from build123d import *

# Parameters (mm, degrees)
SKETCH1_W           = 30
SKETCH1_H           = 30
SKETCH1_R           = 2.65
BOSS_EXTRUDE1_DEPTH = 31
SKETCH2_W           = 30
SKETCH2_H           = 30
BOSS_EXTRUDE2_DEPTH = 10
BOSS_EXTRUDE3_DEPTH = 5
CHAMFER1_SIZE       = 5
CUT_EXTRUDE1_REACH  = 37
SKETCH4_R           = 1.6


with BuildPart() as part:
    # Sketch1 → Boss-Extrude1 (new body)
    with BuildSketch(Plane.XY):
        Rectangle(SKETCH1_W, SKETCH1_H)
        Circle(SKETCH1_R, mode=Mode.SUBTRACT)
    extrude(amount=BOSS_EXTRUDE1_DEPTH)

    # Sketch2 → Boss-Extrude2 (add)
    with BuildSketch(Plane.XY.offset(31)):
        Rectangle(SKETCH2_W, SKETCH2_H)
    extrude(amount=BOSS_EXTRUDE2_DEPTH)

    # Sketch3 → Boss-Extrude3 (add)
    with BuildSketch(Plane(origin=(0, 15, 0), x_dir=(1, 0, 0), z_dir=(0, 1, 0))):
        Polygon((0, 0), (-25, 0), (-25, -50), (25, -50), (25, 0), align=None)
    extrude(amount=BOSS_EXTRUDE3_DEPTH)

    # Chamfer1
    chamfer1_edges = [part.edges().sort_by_distance(p)[0] for p in [
        (15, -15, 20.5),
        (-15, -15, 20.5),
    ]]
    chamfer(chamfer1_edges, length=CHAMFER1_SIZE)

    # Sketch4 → Cut-Extrude1 (cut, up to next)
    with BuildSketch(Plane(origin=(0, 20, 0), x_dir=(1, 0, 0), z_dir=(0, 1, 0)), mode=Mode.PRIVATE) as cut_extrude1_sk1:
        with Locations((-20, -5)):
            Circle(SKETCH4_R)
    cut_extrude1_tool1 = extrude(cut_extrude1_sk1.sketch, amount=-CUT_EXTRUDE1_REACH, mode=Mode.PRIVATE) & part.part
    add(cut_extrude1_tool1.solids().sort_by_distance((-20, 20, 5))[0], mode=Mode.SUBTRACT)
    # Sketch4 → Cut-Extrude1 (cut, up to next)
    with BuildSketch(Plane(origin=(0, 20, 0), x_dir=(1, 0, 0), z_dir=(0, 1, 0)), mode=Mode.PRIVATE) as cut_extrude1_sk2:
        with Locations((20, -5)):
            Circle(SKETCH4_R)
    cut_extrude1_tool2 = extrude(cut_extrude1_sk2.sketch, amount=-CUT_EXTRUDE1_REACH, mode=Mode.PRIVATE) & part.part
    add(cut_extrude1_tool2.solids().sort_by_distance((20, 20, 5))[0], mode=Mode.SUBTRACT)
    # Sketch4 → Cut-Extrude1 (cut, up to next)
    with BuildSketch(Plane(origin=(0, 20, 0), x_dir=(1, 0, 0), z_dir=(0, 1, 0)), mode=Mode.PRIVATE) as cut_extrude1_sk3:
        with Locations((20, -45)):
            Circle(SKETCH4_R)
    cut_extrude1_tool3 = extrude(cut_extrude1_sk3.sketch, amount=-CUT_EXTRUDE1_REACH, mode=Mode.PRIVATE) & part.part
    add(cut_extrude1_tool3.solids().sort_by_distance((20, 20, 45))[0], mode=Mode.SUBTRACT)
    # Sketch4 → Cut-Extrude1 (cut, up to next)
    with BuildSketch(Plane(origin=(0, 20, 0), x_dir=(1, 0, 0), z_dir=(0, 1, 0)), mode=Mode.PRIVATE) as cut_extrude1_sk4:
        with Locations((-20, -45)):
            Circle(SKETCH4_R)
    cut_extrude1_tool4 = extrude(cut_extrude1_sk4.sketch, amount=-CUT_EXTRUDE1_REACH, mode=Mode.PRIVATE) & part.part
    add(cut_extrude1_tool4.solids().sort_by_distance((-20, 20, 45))[0], mode=Mode.SUBTRACT)


solid = part.part
For this review, take the finished solid that the model builds, in its own axes (mm). A direction names the side the tool comes from. Coordinates: 2 decimals unless noted, no trailing zeros. Loops run counter-clockwise (first coordinate to the right, second up) from the corner with the lowest first, then second, coordinate; pieces in that order, holes last. Notation, with made-up numbers: (6, 1) - (38, 1) arc R26 ccw to (38, 34) - close; hole circle Ø7 at (-28, 10.5). An arc over 180 degrees is marked (long way). Return JSON: item names as keys, results as strings.
Item 1: Take a section at D-D (y = 0). Give the boundary of the cut face in (x, z).
Determined:
{"outline": "(-15, 0) - (-2.65, 0) - (-2.65, 31) - (2.65, 31) - (2.65, 0) - (15, 0) - (15, 41) - (-15, 41) - close"}
Item 2: For faces 4 (the flat face through (0, 0, 31)), 5 (the flat face through (0, 0, 41)), 6 (the flat face through (-15, 2, 20)), list the 3-axis set-ups (+Z, -Z, +X, -X, +Y, -Y) from which the entire face can be reached by the end or side of a thin tool; tool diameter is ignored.
Determined:
{"face 4": "-Z", "face 5": "+Z, +X, -X, -Y", "face 6": "+Z, -Z, -X, -Y"}
Item 3: Take a section at A-A (z = 5). Give the boundary of the cut face in (x, y).
Determined:
{"outline": "(-25, 15) - (-21.6, 15) - (-21.6, 20) - (-25, 20) - close; (-18.4, 15) - (-15, 15) - (-15, -10) - (-10, -15) - (10, -15) - (15, -10) - (15, 15) - (18.4, 15) - (18.4, 20) - (-18.4, 20) - close; (21.6, 15) - (25, 15) - (25, 20) - (21.6, 20) - close; hole circle Ø5.3 at (0, 0)"}
Item 4: For line 1 (X direction, y = 17.8, z = 5); line 2 (Z direction, x = -20, y = 16.85); line 3 (Z direction, x = 1, y = 11), list the stretches that pass through material, from the lowest coordinate up.
Determined:
{"line 1": "x = -25 to -21.6, -18.4 to 18.4, 21.6 to 25", "line 2": "z = 0 to 3.4, 6.6 to 43.4, 46.6 to 50", "line 3": "z = 0 to 41"}
Item 5: Take a section at C-C (z = 23.5). Give the boundary of the cut face in (x, y), then the cut area to 3 significant figures.
Determined:
{"outline": "(-25, 15) - (-15, 15) - (-15, -10) - (-10, -15) - (10, -15) - (15, -10) - (15, 15) - (25, 15) - (25, 20) - (-25, 20) - close; hole circle Ø5.3 at (0, 0)", "area": "1,100 mm2"}
Item 6: Mouldability with a two-part tool opening along Z and no side actions: class faces 1 (the flat face through (0, 17, 50)), 2 (the cylindrical face through (18.73, 17.54, 45.97)), 3 (the flat face through (-25, 17, 25)) as pulls with the +Z half, pulls with the -Z half, needs draft (parallel to the pull), parting line crosses it, or undercut.
Determined:
{"face 1": "pulls with the +Z half", "face 2": "undercut", "face 3": "needs draft"}
Item 7: Take a section at B-B (x = 20). Give the boundary of the cut face in (y, z), then the cut area to 3 significant figures.
Determined:
{"outline": "(15, 0) - (20, 0) - (20, 3.4) - (15, 3.4) - close; (15, 6.6) - (20, 6.6) - (20, 43.4) - (15, 43.4) - close; (15, 46.6) - (20, 46.6) - (20, 50) - (15, 50) - close", "area": "218 mm2"}
Item 8: Insertion check: pin 1 (4 mm diameter, centred on x = -13.5, y = 2.5, fed in from +Z); pin 2 (4 mm diameter, centred on y = 12.5, z = 30, fed in from +X); pin 3 (1.9 mm diameter, centred on x = -20, z = 5, fed in from -Y); pin 4 (4 mm diameter, centred on x = 20, z = 5, fed in from -Y). Each pin has a flat end and moves straight along its axis. Give the tip position at first contact, or say it passes through.
Determined:
{"pin 1": "stops at z = 41", "pin 2": "stops at x = 15", "pin 3": "passes through", "pin 4": "stops at y = 15"}
